The listing builds one solid part. Answer for the finished solid, in the listing's coordinates (mm). A direction names the side the tool comes from. Give positions to 0.01 mm unless a question says otherwise; leave off trailing zeros. Order: outer loops, then holes, each group sorted by start corner. A loop starts at its lowest first (then second) coordinate and runs counter-clockwise, first axis right, second up. Notation, with made-up numbers: M -9.75,76.5 L 2.25,76.5 A26 cw 2.25,93.5 Z; hole C -23,48 d2. An arc over 180 degrees is marked long. Answer as a JSON object with one key per item and string values. Group by question number.
```python
from build123d import *

# Parameters (mm, degrees)
BOSS_EXTRUDE1_DEPTH = 9.525
SKETCH4_R           = 6.35
BOSS_EXTRUDE2_DEPTH = 25.4
SKETCH5_R           = 6.35
BOSS_EXTRUDE3_DEPTH = 25.4
SKETCH6_R           = 3.175
CUT_EXTRUDE1_DEPTH  = 19.05
SKETCH7_W           = 19.05
SKETCH7_H           = 25.4
BOSS_EXTRUDE4_DEPTH = 5.08
SKETCH8_R           = 3.81
CUT_EXTRUDE2_DEPTH  = 6.35


with BuildPart() as part:
    # Sketch2 → Boss-Extrude1 (new, symmetric)
    with BuildSketch(Plane(origin=(0, 0, 0), x_dir=(0, 0, -1), z_dir=(1, 0, 0))):
        with BuildLine():
            Line((-158.75, 12.7), (158.75, 12.7))
            ThreePointArc((158.75, 12.7), (171.45, 0), (158.75, -12.7))
            Line((158.75, -12.7), (-158.75, -12.7))
            ThreePointArc((-158.75, -12.7), (-171.45, 0), (-158.75, 12.7))
        make_face()
    extrude(amount=BOSS_EXTRUDE1_DEPTH, both=True)

    # Sketch4 → Boss-Extrude2 (add)
    with BuildSketch(Plane.ZY.offset(9.525)):
        with Locations((157.48, 0)):
            Circle(SKETCH4_R)
    extrude(amount=BOSS_EXTRUDE2_DEPTH)

    # Sketch5 → Boss-Extrude3 (add)
    with BuildSketch(Plane(origin=(9.525, 0, 0), x_dir=(0, 0, -1), z_dir=(1, 0, 0))):
        with Locations(Location((157.48, 0, 0), (0, 0, 180))):
            Circle(SKETCH5_R)
    extrude(amount=BOSS_EXTRUDE3_DEPTH)

    # Sketch6 → Cut-Extrude1 (cut)
    with BuildSketch(Plane(origin=(9.525, 0, 0), x_dir=(0, 0, -1), z_dir=(1, 0, 0))):
        with Locations((-65.6082, 0)):
            Circle(SKETCH6_R)
    extrude(amount=-CUT_EXTRUDE1_DEPTH, mode=Mode.SUBTRACT)

    # Sketch7 → Boss-Extrude4 (add)
    with BuildSketch(Plane.XZ.offset(12.7)):
        with Locations((0, -60.452)):
            Rectangle(SKETCH7_W, SKETCH7_H)
    extrude(amount=BOSS_EXTRUDE4_DEPTH)

    # Sketch8 → Cut-Extrude2 (cut, symmetric)
    with BuildSketch(Plane(origin=(0, 0, 0), x_dir=(1, 0, 0), z_dir=(0, 1, 0))):
        with Locations(Location((-28.575, -157.48, 0), (0, 0, 270))):
            Circle(SKETCH8_R)
        with Locations(Location((28.575, 157.48, 0), (0, 0, 270))):
            Circle(SKETCH8_R)
    extrude(amount=CUT_EXTRUDE2_DEPTH, both=True, mode=Mode.SUBTRACT)


solid = part.part
```
Item 1: Section A-A (x = 6.5) is taken. Determine the outline of the cut face in (y, z) (3 decimals).
Item 2: Flat-ended cylindrical pins translate along their axes: P1, Ø21, axis at x = -4.5, z = 47.5, coming from the -Y side; P2, Ø6, axis at y = -13.5, z = 9, coming from the -X side (3 decimals); P3, Ø1.5, axis at x = 0, y = -14.5, coming from the +Z side. Find the tip coordinate at first contact, or state that the pin passes through.
Item 3: Consider probe 1 along X at (y, z) = (4, 157) (3 decimals); probe 2 along Y at (x, z) = (1, 60); probe 3 along X at (y, z) = (-2, -45) (3 decimals). Determine where each line is inside the solid, lowest interval first. Write a range as from..to.
Item 4: A tool of negligible diameter and unlimited length cuts with its end or side. For faces 4 (the flat face through (0, -12.7, 54)), 5 (the cylindrical face through (-22.047, 0.279, 151.136)), 6 (the cylindrical face through (0.133, 0.279, -171.447)), from which of +Z, -Z, +X, -X, +Y, -Y can it reach the whole face along a straight path? Write none if from no direction.
Item 5: Determine the mould class of faces 1 (the cylindrical face through (28.743, 0.089, -161.286)), 2 (the cylindrical face through (22.047, -0.279, -163.824)), 3 (the flat face through (0, -12.7, -117)) for opening direction Z: released by +Z, released by -Z, zero draft, split by the parting line, or undercut.
Item 6: Section B-B (z = -110) is taken. Determine the outline of the cut face in (x, y) (3 decimals).
Values found:
{
 "1": {"outline": "M -17.78,-73.152 L -12.7,-73.152 L -12.7,-158.75 A12.7 ccw 12.7,-158.75 L 12.7,158.75 A12.7 ccw -12.7,158.75 L -12.7,-47.752 L -17.78,-47.752 Z; hole C 0,65.608 d6.35"},
 "2": {"P1": "stops at y = -12.7", "P2": "stops at x = -9.525", "P3": "stops at z = -47.75"},
 "3": {"probe 1": "x = -34.925..-32.355, -24.795..9.525", "probe 2": "y = -12.7..12.7", "probe 3": "x = -9.525..9.525"},
 "4": {"face 4": "+Z, +X, -X, -Y", "face 5": "-X", "face 6": "-Z, +X, -X"},
 "5": {"face 1": "undercut", "face 2": "split by the parting line", "face 3": "zero draft"},
 "6": {"outline": "M -9.525,-12.7 L 9.525,-12.7 L 9.525,12.7 L -9.525,12.7 Z"}
}
